Can you work these out from the drawing? Everything is in mm from the part's minimum corner. A direction names the side the tool comes from. Give positions to 0.01 mm unless a question says otherwise; leave off trailing zeros. Loops run counter-clockwise (first coordinate to the right, second up) from the corner with the lowest first, then second, coordinate; pieces in that order, holes last. Notation, with made-up numbers: (-28.5, 70.5) - (-20.5, 70.5) arc R36 cw to (-20.5, 106.5) - close; hole circle Ø11 at (30.25, -13.75). An arc over 180 degrees is marked (long way). Answer in a Markdown table with one row per item. Add a question column.
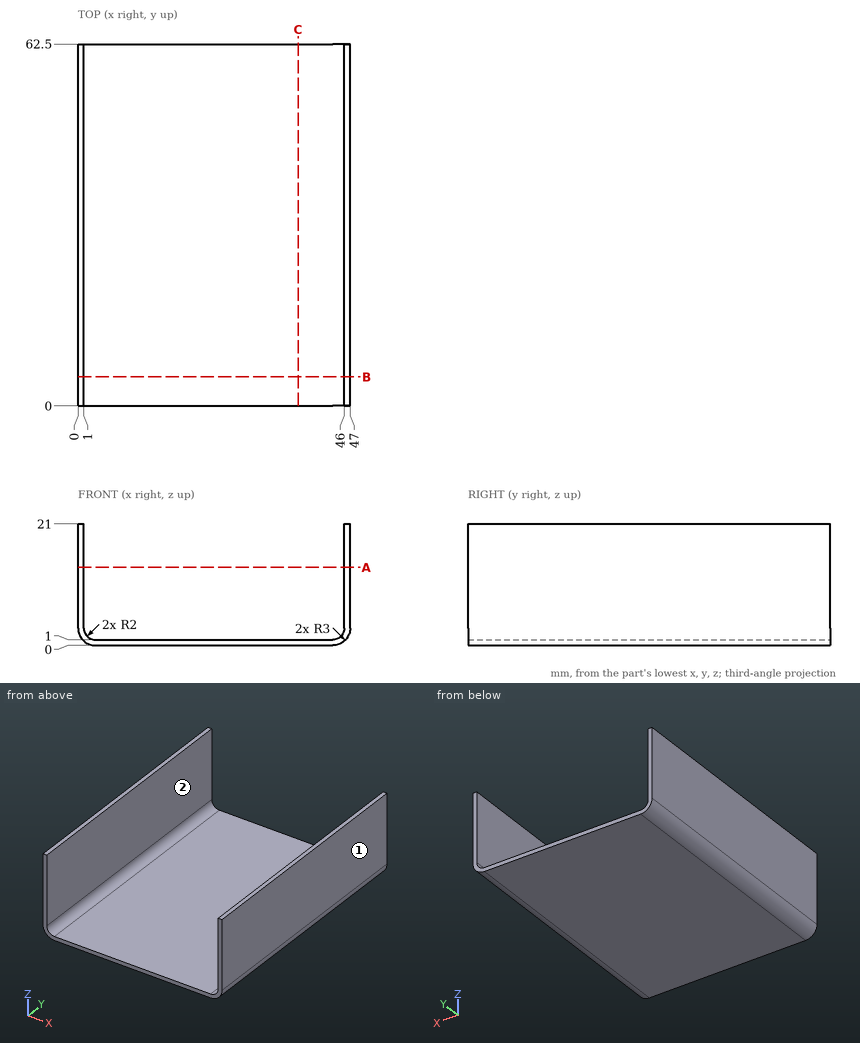
(1) I want a section at A-A on z = 13.5. Please give me the cut outline in (x, y), then the cut area to 3 significant figures.
(2) I want a section at B-B on y = 5. Please give me the cut outline in (x, z), then the cut area to 3 significant figures.
(3) Please list where these lines run through material, in increasing order: line 1 (X direction, y = 20.5, z = 11); line 2 (Z direction, x = 6, y = 47); line 3 (X direction, y = 25.5, z = 2.5).
(4) For pin 1 Ø3 at (x, y) = (21, 37.5) entering from +Z, with a flat end and sliding along its axis, tell me the tip position at first contact or that it passes through.
(5) I want a section at C-C on x = 38. Please give me the cut outline in (y, z).
(6) On a 3-axis mill with a long thin cutter (end or side, diameter ignored), from which of +Z, -Z, +X, -X, +Y, -Y can I reach the whole of each face in a straight line? I mean the marked faces 1 and 2. Say none if no direction works.
Reported:
| question | item | result |
|---|---|---|
| 1 | outline | (0, 0) - (1, 0) - (1, 62.5) - (0, 62.5) - close; (46, 0) - (47, 0) - (47, 62.5) - (46, 62.5) - close |
| 1 | area | 125 mm² |
| 2 | outline | (0, 3) arc R3 ccw to (3, 0) - (44, 0) arc R3 ccw to (47, 3) - (47, 21) - (46, 21) - (46, 3) arc R2 cw to (44, 1) - (3, 1) arc R2 cw to (1, 3) - (1, 21) - (0, 21) - close |
| 2 | area | 84.9 mm² |
| 3 | line 1 | 0 to 1, 46 to 47 |
| 3 | line 2 | 0 to 1 |
| 3 | line 3 | 0.04 to 1.06, 45.94 to 46.96 |
| 4 | pin 1 | z = 1 |
| 5 | outline | (0, 0) - (62.5, 0) - (62.5, 1) - (0, 1) - close |
| 6 | face 1 | +Z, -Z, +X, +Y, -Y |
| 6 | face 2 | +Z, +Y, -Y |
